```python
from build123d import *

# Parameters (mm, degrees)
SKETCH_W            = 10.15
SKETCH_H            = 10.15
PAD_DEPTH           = 5.5
PAD001_DEPTH        = 5.5
SKETCH003_R         = 0.5
PAD003_DEPTH        = 20
LINEARPATTERN_COUNT = 7
LINEARPATTERN_PITCH = 10.15


with BuildPart() as part:
    # Sketch → Pad (new body)
    with BuildSketch(Plane.XY):
        Rectangle(SKETCH_W, SKETCH_H)
    pad = extrude(amount=PAD_DEPTH)

    # Sketch001 (on Face6 of Pad) → Pad001 (join)
    with BuildSketch(Plane.XY.offset(5.5)):
        Polygon((-5.075, 2.575), (-2.575, 5.075), (-5.075, 5.075), align=None)
        Polygon((2.575, -5.075), (5.075, -5.075), (5.075, -2.575), align=None)
    pad001 = extrude(amount=PAD001_DEPTH)

    # Sketch003 (on Face4 of Pad001) → Pad003 (join)
    with BuildSketch(Plane(origin=(0, 0, 0), x_dir=(1, 0, 0), z_dir=(0, 0, -1))):
        with Locations((1.6, 3.5)):
            Circle(SKETCH003_R)
        with Locations((-1.6, -3.5)):
            Circle(SKETCH003_R)
    pad003 = extrude(amount=PAD003_DEPTH)

    # LinearPattern: Pad, Pad001, Pad003 ×7
    with Locations(*[(i * LINEARPATTERN_PITCH, 0, 0) for i in range(1, LINEARPATTERN_COUNT)]):
        add(pad)
        add(pad001)
        add(pad003)


with BuildPart() as part_1:
    # Body placement: moved
    add(part.part.moved(Location((0, 0, 16.5))))


solid = part_1.part
```
Check sheet for the modelled part. Datum: model origin and axes. Units: mm. A direction names the side the tool comes from. Round coordinates to 2 decimals unless told otherwise and drop trailing zeros. Loops run counter-clockwise (first coordinate to the right, second up) from the corner with the lowest first, then second, coordinate; pieces in that order, holes last. Notation, with made-up numbers: (47, 46.25) - (61, 46.25) arc R25 cw to (61, 76.25) - close; hole circle Ø4 at (-27, 7). An arc over 180 degrees is marked (long way). Answer as a JSON object with one key per item and string values. Group by question number.
Q1. Gauge pin test, flat ends, axial feed: P1, Ø5, axis at y = 4, z = 5, coming from the -X side; P2, Ø5, axis at x = 3, z = 7.5, coming from the -Y side; P3, Ø3, axis at x = 44, y = 1.5, coming from the -Z side. Record the tip position at first contact, or that the pin passes through.
Q2. Mould release check, pull along X, two halves, no side actions. Record for faces 4 (the face through (64.74, -3.81, 24.71)), 5 (the face through (26, 4, 27.5)), 6 (the face through (65.975, -1, 21)): released by +X, released by -X, zero draft, split by the parting line, or undercut.
Q3. Set-up check for faces 1 (the face through (15, -4, 27.5)), 2 (the face through (46.9, 3.8, 24.7)), 3 (the face through (15.225, 4, 25)): record each of +Z, -Z, +X, -X, +Y, -Y from which the full face is reachable in a straight line by a thin tool's end or side.
Q4. Sectioned sample at A-A, the plane z = 5. Count the separate pieces of the cut face and the enclosed holes in it, plus the area to 3 significant figures.
Q5. Sectioned sample at B-B, the plane y = -0.5. Enter the section's corners in (x, z) (3 decimals), plus the area to 3 significant figures.
Q6. Scan lines: line 1 along Z through (x, y) = (51, 1.75); line 2 along Y through (x, z) = (39, 12); line 3 along Y through (x, z) = (35, 25) (3 decimals). Record each from-to range of solid material in increasing order. Write a range as [from, to].
Solution:
{
 "1": {"P1": "stops at x = -2.1", "P2": "stops at y = -4", "P3": "stops at z = 16.5"},
 "2": {"face 4": "undercut", "face 5": "zero draft", "face 6": "released by +X"},
 "3": {"face 1": "+Z, +X, -X, +Y, -Y", "face 2": "+Z, -Y", "face 3": "+Z, +Y"},
 "4": {"separate pieces": "14", "enclosed holes": "0", "area": "11.0 mm²"},
 "5": {"outline": "(-5.075, 16.5) - (65.975, 16.5) - (65.975, 22) - (-5.075, 22) - close", "area": "391 mm²"},
 "6": {"line 1": "z = [16.5, 22]", "line 2": "y = [3, 4]", "line 3": "y = [-5.075, -3.1]"}
}
